```python
from build123d import *

# Parameters (mm, degrees)
FILLET1_R = 0.0635


with BuildPart() as part:
    # Sketch1 → Revolve1 (revolve)
    with BuildSketch(Plane(origin=(0, 0, 0), x_dir=(0, 0, -1), z_dir=(1, 0, 0))):
        Polygon((0, 2.99085), (9.2202, 2.99085), (9.2202, 1.397), (10.8204, 1.397), (10.8204, 0.5), (13.6144, 0.5), (13.6144, 0), (1.27, 0), (1.27, 1.84785), (0, 1.84785), align=None)
    revolve(axis=Axis((0, 0, 14.404430618), (0, 0, -1)))

    # Fillet1
    fillet1_edges = [part.edges().sort_by_distance(p)[0] for p in [
        (0, -2.99085, 0),
        (0, -2.99085, -9.2202),
    ]]
    fillet(fillet1_edges, radius=FILLET1_R)


solid = part.part
```
Geometry check sheet. Reference: the model listing, model coordinates, mm. A direction names the side the tool comes from. Round coordinates to 2 decimals unless told otherwise and drop trailing zeros. Loops run counter-clockwise (first coordinate to the right, second up) from the corner with the lowest first, then second, coordinate; pieces in that order, holes last. Notation, with made-up numbers: (33.5, 55) -> (60.5, 55) arc R20 cw to (60.5, 70) -> close; hole circle Ø5 at (46, -14.5). An arc over 180 degrees is marked (long way). Use a Markdown table: item, result.
(1) Set-up check for faces 5 (the flat face through (0, 0, -13.614)), 6 (the cylindrical face through (-0.85, -1.11, -10.03)): record each of +Z, -Z, +X, -X, +Y, -Y from which the full face is reachable in a straight line by a thin tool's end or side.
Calculated:
| item | result |
|---|---|
| face 5 | -Z, +X, -X, +Y, -Y |
| face 6 | -Z |
(2) Sectioned sample at D-D (z = -5.5). Enter the section's corners in (x, y), then the cut area to 3 significant figures.
Calculated:
| item | result |
|---|---|
| outline | circle Ø5.98 at (0, 0) |
| area | 28.1 mm² |
(3) Scan lines: probe 1 along X at (y, z) = (0, -0.45); probe 2 along Z at (x, y) = (1.1, 0.9); probe 3 along Z at (x, y) = (1.7, 1.75). Record each from-to range of solid material in increasing order.
Calculated:
| item | result |
|---|---|
| probe 1 | -2.99 to -1.85, 1.85 to 2.99 |
| probe 2 | -9.22 to -1.27 |
| probe 3 | -9.22 to 0 |
(4) Mould release check, pull along Y, two halves, no side actions. Record for faces 1 (the flat face through (0, 0, -1.27)), 2 (the flat face through (0, 1, -10.82)), 3 (the cylindrical face through (-1.804, -0.401, -0.626)), 4 (the cylindrical face through (-0.488, -0.108, -12.237)): released by +Y, released by -Y, zero draft, split by the parting line, or undercut.
Calculated:
| item | result |
|---|---|
| face 1 | undercut |
| face 2 | zero draft |
| face 3 | undercut |
| face 4 | split by the parting line |
(5) Sectioned sample at C-C (z = -12). Enter the section's corners in (x, y).
Calculated:
| item | result |
|---|---|
| outline | circle Ø1 at (0, 0) |
(6) Sectioned sample at A-A (x = 0). Enter the section's corners in (y, z), then the cut area to 3 significant figures.
Calculated:
| item | result |
|---|---|
| outline | (-2.99, -9.16) arc R0.06 ccw to (-2.93, -9.22) -> (-1.4, -9.22) -> (-1.4, -10.82) -> (-0.5, -10.82) -> (-0.5, -13.61) -> (0.5, -13.61) -> (0.5, -10.82) -> (1.4, -10.82) -> (1.4, -9.22) -> (2.93, -9.22) arc R0.06 ccw to (2.99, -9.16) -> (2.99, -0.06) arc R0.06 ccw to (2.93, 0) -> (1.85, 0) -> (1.85, -1.27) -> (-1.85, -1.27) -> (-1.85, 0) -> (-2.93, 0) arc R0.06 ccw to (-2.99, -0.06) -> close |
| area | 57.7 mm² |
(7) Go/stop test with flat-tipped pins: P1, Ø1, axis at x = -2, z = -6.5, coming from the +Y side; P2, Ø2, axis at y = 2, z = -8.5, coming from the +X side; P3, Ø1, axis at y = 0, z = -12, coming from the +X side. Record where each tip stops, or that it passes through.
Calculated:
| item | result |
|---|---|
| P1 | y = 2.59 |
| P2 | x = 2.82 |
| P3 | x = 0.5 |
